Source: CAD feature listing. Evaluate the final solid. Frame: model axes, mm. A direction names the side the tool comes from. Round coordinates to 2 decimals unless told otherwise and drop trailing zeros. Write each loop counter-clockwise with the first axis right and the second up, starting at its lowest first coordinate (ties: lowest second). Pieces come first, ordered by that corner, then holes.
from build123d import *

# Parameters (mm, degrees)
F1_DEPTH = 457.2
F3_DEPTH = 2.794


with BuildPart() as f1:
    # F0 (on Top) → F1 (new body)
    with BuildSketch(Plane.XY):
        with BuildLine():
            ThreePointArc((0, 5.969), (1.74828, 1.74828), (5.969, 0))
            Line((5.969, 0), (19.431, 0))
            ThreePointArc((19.431, 0), (23.65172, 1.74828), (25.4, 5.969))
            Line((25.4, 5.969), (25.4, 19.431))
            ThreePointArc((25.4, 19.431), (23.65172, 23.65172), (19.431, 25.4))
            Line((19.431, 25.4), (5.969, 25.4))
            ThreePointArc((5.969, 25.4), (1.74828, 23.65172), (0, 19.431))
            Line((0, 19.431), (0, 5.969))
        make_face()
        with BuildLine():
            ThreePointArc((2.794, 19.431), (3.723936, 21.676064), (5.969, 22.606))
            Line((5.969, 22.606), (19.431, 22.606))
            ThreePointArc((19.431, 22.606), (21.676064, 21.676064), (22.606, 19.431))
            Line((22.606, 19.431), (22.606, 5.969))
            ThreePointArc((22.606, 5.969), (21.676064, 3.723936), (19.431, 2.794))
            Line((19.431, 2.794), (5.969, 2.794))
            ThreePointArc((5.969, 2.794), (3.723936, 3.723936), (2.794, 5.969))
            Line((2.794, 5.969), (2.794, 19.431))
        make_face(mode=Mode.SUBTRACT)
    extrude(amount=F1_DEPTH)

    # F2 (on face) → F3 (cut, through all)
    with BuildSketch(Plane(origin=(0, 25.4, 0), x_dir=(-1, 0, 0), z_dir=(0, 1, 0))):
        with BuildLine():
            ThreePointArc((-8.636, 381), (-9.826318, 383.873682), (-12.7, 385.064))
            ThreePointArc((-12.7, 385.064), (-15.573682, 378.126318), (-8.636, 381))
        make_face()
    extrude(amount=-F3_DEPTH, mode=Mode.SUBTRACT)


solid = f1.part
1) Material intervals for line 1 (X direction, y = 16.25, z = 107); line 2 (Z direction, x = 12.7, y = 24.55), sorted ascending.
Taken from the geometry:
line 1: x = 0 to 2.79, 22.61 to 25.4
line 2: z = 0 to 376.94, 385.06 to 457.2
2) Section query B-B on z = 43.5. Return the cut outline in (x, y) (3 decimals), then the cut area to 3 significant figures.
Taken from the geometry:
outline: (0, 5.969) arc R5.969 ccw to (5.969, 0) - (19.431, 0) arc R5.969 ccw to (25.4, 5.969) - (25.4, 19.431) arc R5.969 ccw to (19.431, 25.4) - (5.969, 25.4) arc R5.969 ccw to (0, 19.431) - close; hole (2.794, 5.969) arc R3.175 ccw to (5.969, 2.794) - (19.431, 2.794) arc R3.175 ccw to (22.606, 5.969) - (22.606, 19.431) arc R3.175 ccw to (19.431, 22.606) - (5.969, 22.606) arc R3.175 ccw to (2.794, 19.431) - close
area: 231 mm2
3) Reachability of faces 1 (the face through (13, 25.4, 225)), 2 (the face through (13, 2.794, 225)) from +Z, -Z, +X, -X, +Y, -Y: full face, straight path, thin tool, end or side. Return the list, or none.
Taken from the geometry:
face 1: +Z, -Z, +X, -X, +Y
face 2: +Z, -Z
4) Pull-direction query (Y, two-part tool) for faces 3 (the face through (13, 2, 0)), 4 (the face through (13, 22.606, 225)), 5 (the face through (13, 0, 225)); classes: released by +Y, released by -Y, zero draft, split by the parting line, or undercut.
Taken from the geometry:
face 3: zero draft
face 4: undercut
face 5: released by -Y
5) Section query A-A on y = 12.5. Return the cut outline in (x, z).
Taken from the geometry:
outline: (0, 0) - (2.79, 0) - (2.79, 457.2) - (0, 457.2) - close; (22.61, 0) - (25.4, 0) - (25.4, 457.2) - (22.61, 457.2) - close
